Part print with two shaded views. Sizes in mm from the minimum x, y, z corner. Give positions to 0.01 mm unless a question says otherwise; leave off trailing zeros. Write each loop counter-clockwise with the first axis right and the second up, starting at its lowest first coordinate (ties: lowest second). Pieces come first, ordered by that corner, then holes. Notation, with made-up numbers: (-33.5, -6.5) - (-23.5, -6.5) arc R14 cw to (-23.5, 12.5) - close; hole circle Ø5 at (68.25, -17). An arc over 180 degrees is marked (long way). One line per item, written item: value. Start each with the question number.
(1) Cut at A-A, the plane z = 30. List the corners of the cut face in (x, y).
(2) Drop flat-ended pins along their axis: P1, Ø5, axis at x = 5, z = 9.5, coming from the +Y side; P2, Ø18, axis at y = 30, z = 30, coming from the -X side; P3, Ø2, axis at x = 21.5, z = 14, coming from the +Y side. Give the stop position or say it passes through.
(3) Cut at C-C, the plane y = 638. List the corners of the cut face in (x, z), and give its area (3 significant figures).
(4) Probe L1, parallel to Z at x = 5, y = 638; L2, parallel to Y at x = 12, z = 27; L3, parallel to Y at x = 10.75, z = 33.5. List the from-to ranges inside material, lowest first.
(5) Cut at B-B, the plane x = 9.5. List the corners of the cut face in (y, z).
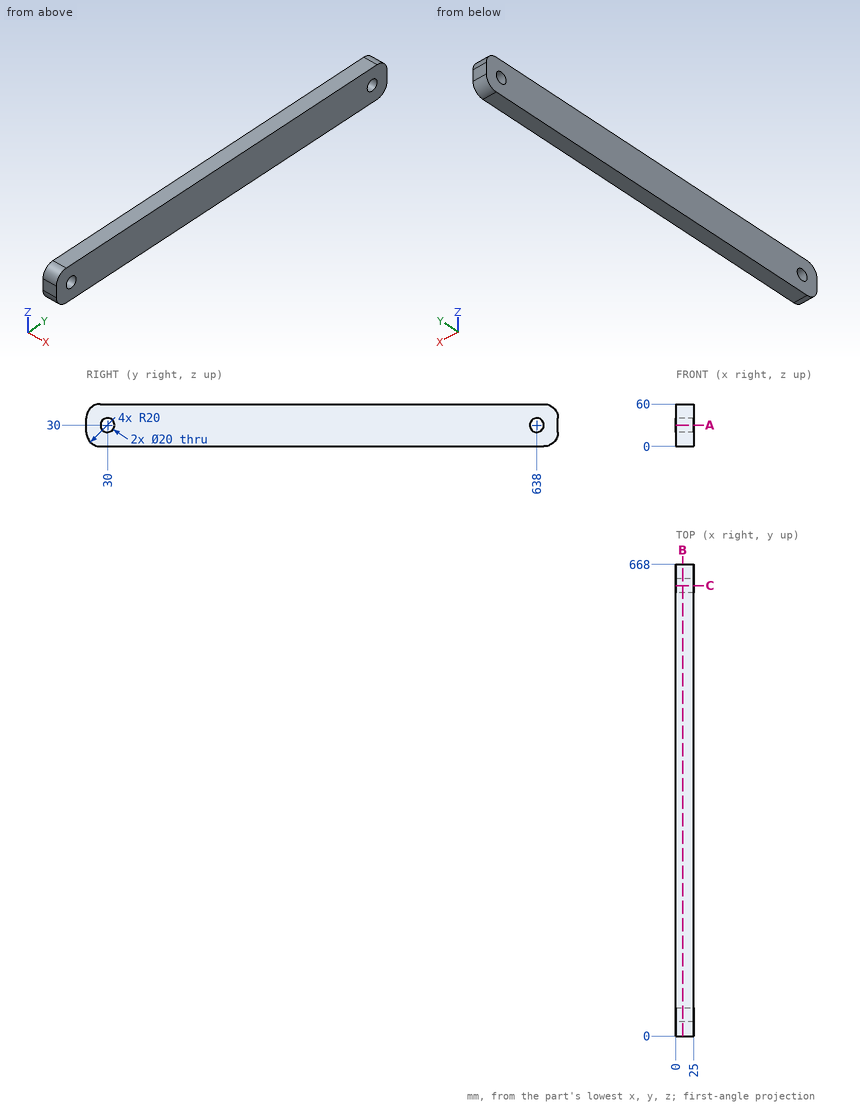
Answers follow:
1. outline: (0, 0) - (25, 0) - (25, 20) - (0, 20) - close; (0, 40) - (25, 40) - (25, 628) - (0, 628) - close; (0, 648) - (25, 648) - (25, 668) - (0, 668) - close
2. P1: stops at y = 666.33
2. P2: passes through
2. P3: stops at y = 667.36
3. outline: (0, 0) - (25, 0) - (25, 20) - (0, 20) - close; (0, 40) - (25, 40) - (25, 60) - (0, 60) - close
3. area: 1,000 mm²
4. L1: z = 0 to 20, 40 to 60
4. L2: y = 0 to 20.46, 39.54 to 628.46, 647.54 to 668
4. L3: y = 0 to 20.63, 39.37 to 628.63, 647.37 to 668
5. outline: (0, 20) arc R20 ccw to (20, 0) - (648, 0) arc R20 ccw to (668, 20) - (668, 40) arc R20 ccw to (648, 60) - (20, 60) arc R20 ccw to (0, 40) - close; hole circle Ø20 at (30, 30); hole circle Ø20 at (638, 30)
